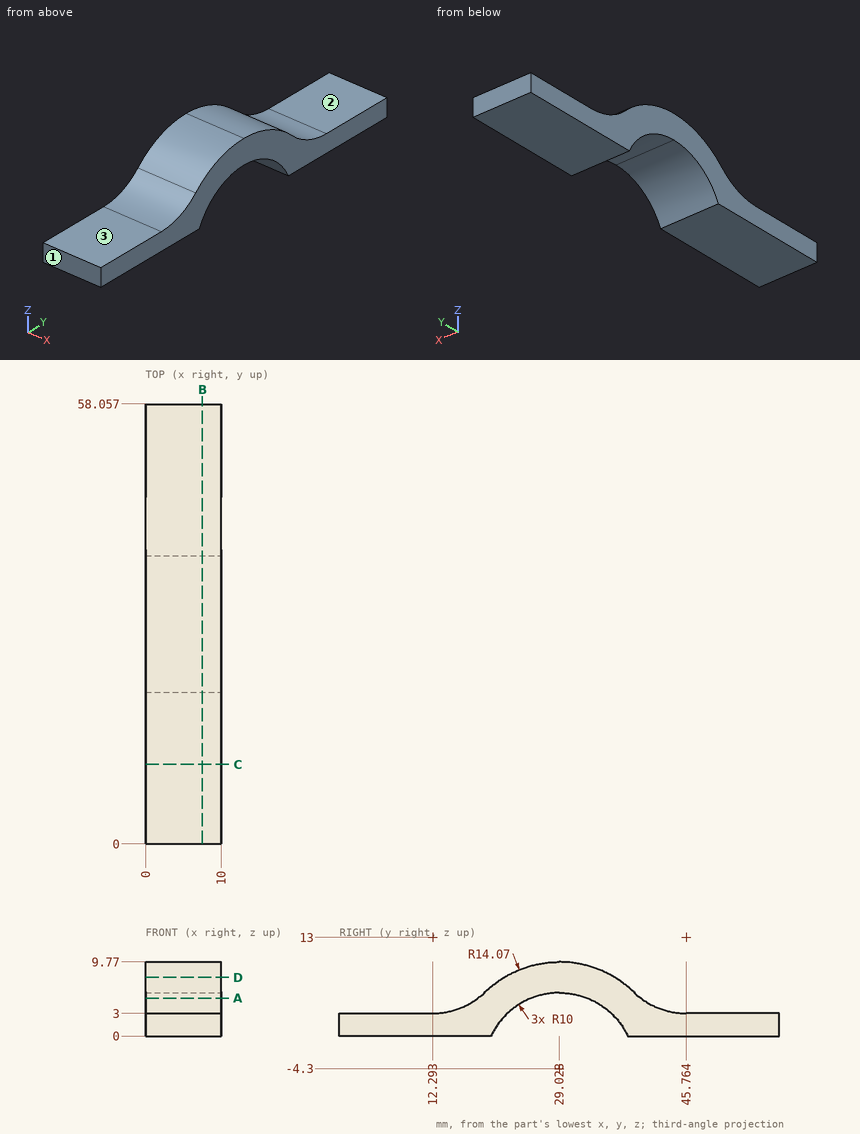
Here's the drawing with two shaded views (mm, measured from the low corner). I have some questions. A direction names the side the tool comes from. Round coordinates to 2 decimals unless told otherwise and drop trailing zeros. Loops run counter-clockwise (first coordinate to the right, second up) from the corner with the lowest first, then second, coordinate; pieces in that order, holes last. Notation, with made-up numbers: M -5.75,49 L 20.25,49 A15 ccw 20.25,73 Z; hole C -31.75,-21.5 d8. An arc over 180 degrees is marked long. Put each result on its own line as item: value.
Q1. Imagine slicing it at C-C (y = 10.5). Write out the boundary of the cut face in (x, z).
Check result:
outline: M 0,0 L 10,0 L 10,3 L 0,3 Z
Q2. Imagine slicing it at D-D (z = 7.75). Write out the boundary of the cut face in (x, y) (1 decimal), then the cut area to 3 significant figures.
Check result:
outline: M 0,21.8 L 10,21.8 L 10,36.3 L 0,36.3 Z
area: 145 mm2
Q3. I need wall thicknesses on probe 1 along Z at (x, y) = (5, 49); probe 2 along Y at (x, z) = (8.5, 1.25) (1 decimal); probe 3 along Y at (x, z) = (1.25, 1.75) (1 decimal). Which ranges of each line are inside material? Lowest first, please.
Check result:
probe 1: 0 to 3
probe 2: 0 to 20.7, 37.3 to 58.1
probe 3: 0 to 21.1, 37 to 58.1
Q4. Imagine slicing it at A-A (z = 5). Write out the boundary of the cut face in (x, y), then the cut area to 3 significant figures.
Check result:
outline: M 0,18.29 L 10,18.29 L 10,25.35 L 0,25.35 Z; M 0,32.7 L 10,32.7 L 10,39.76 L 0,39.76 Z
area: 141 mm2
Q5. Imagine slicing it at B-B (x = 7.5). Write out the boundary of the cut face in (y, z) (1 decimal), then the cut area to 3 significant figures.
Check result:
outline: M 0,0 L 20,0 A10 cw 38.1,0 L 58.1,0 L 58.1,3 L 45.8,3 A10 cw 38.8,5.8 A14.1 ccw 19.2,5.8 A10 cw 12.3,3 L 0,3 Z
area: 221 mm2
Q6. For pin 1 (3 mm diameter, centred on x = 2, z = 7, fed in from +Y); pin 2 (1.5 mm diameter, centred on x = 4.5, z = 6.5, fed in from -Y); pin 3 (5 mm diameter, centred on x = 5, y = 5, fed in from +Z), each with a flat end and sliding along its axis, tell me the tip position at first contact or that it passes through.
Check result:
pin 1: y = 39.15
pin 2: y = 19.18
pin 3: z = 3
Q7. On a 3-axis mill with a long thin cutter (end or side, diameter ignored), from which of +Z, -Z, +X, -X, +Y, -Y can I reach the whole of each face in a straight line? I mean the marked faces 1, 2 and 3. Say none if no direction works.
Check result:
face 1: +Z, -Z, +X, -X, -Y
face 2: +Z, +X, -X, +Y
face 3: +Z, +X, -X, -Y
